The listing builds one solid part. Answer for the finished solid, in the listing's coordinates (mm). Face numbers are marked on the shaded views. Round coordinates to 2 decimals unless told otherwise and drop trailing zeros. Write each loop counter-clockwise with the first axis right and the second up, starting at its lowest first coordinate (ties: lowest second). Pieces come first, ordered by that corner, then holes.
Item 1: Each of these flat-tipped pins is pushed along its axis until it touches: pin 1 (1.5 mm diameter, centred on y = 12.5, z = 15, fed in from -X); pin 2 (3 mm diameter, centred on x = -8, z = -44.5, fed in from +Y); pin 3 (12 mm diameter, centred on x = 11, z = 60.5, fed in from +Y). Where does it stop, or does it pass through?
Item 2: For a pull along X with two mould halves and no side action, classify the marked faces 1 and 2 as +X half, -X half, draft (parallel to the pull), parting line (faces both ways), or undercut.
Item 3: Find section A-A on x = 0. Give the vertices of the cut face in (y, z), then the cut area to 3 significant figures.
Item 4: Find the intervals of material crossed by probe 1 along Z at (x, y) = (0, 13); probe 2 along Y at (x, z) = (0, 21); probe 3 along Z at (x, y) = (-1.5, 12), in increasing order.
Item 5: Find section C-C on z = -13. Give the vertices of the cut face in (x, y).
Item 6: Find section D-D on y = -4. Give the vertices of the cut face in (x, z).
Item 7: Find section B-B on y = 3.5. Give the vertices of the cut face in (x, z).
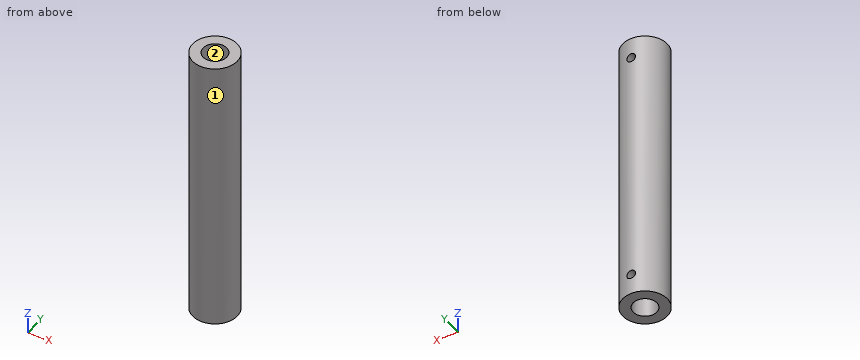
```python
from build123d import *

# Parameters (mm, degrees)
SKETCH2_R                = 16
SKETCH2_R_2              = 8.5
BOSS_EXTRUDE1_DEPTH      = 100
BOSS_EXTRUDE1_DEPTH_BACK = 100
SKETCH4_R                = 3.1
CUT_EXTRUDE1_DEPTH       = 17


with BuildPart() as part:
    # Sketch2 → Boss-Extrude1 (new body, two sides)
    with BuildSketch(Plane.XY) as boss_extrude1_sk:
        Circle(SKETCH2_R)
        Circle(SKETCH2_R_2, mode=Mode.SUBTRACT)
    extrude(amount=BOSS_EXTRUDE1_DEPTH)
    extrude(boss_extrude1_sk.sketch, amount=-BOSS_EXTRUDE1_DEPTH_BACK)

    # Sketch4 → Cut-Extrude1 (cut, through all)
    with BuildSketch(Plane(origin=(0, 0, 0), x_dir=(1, 0, 0), z_dir=(0, 1, 0))):
        with Locations((0, -85)):
            Circle(SKETCH4_R)
    cut_extrude1 = extrude(amount=CUT_EXTRUDE1_DEPTH, mode=Mode.SUBTRACT)

    # Mirror1: Cut-Extrude1 across plane
    add(cut_extrude1.mirror(Plane.XY), mode=Mode.SUBTRACT)


solid = part.part
```
Check values:
1. pin 1: stops at x = -10.86
1. pin 2: stops at y = 14.62
1. pin 3: stops at y = 15.2
2. face 1: parting line
2. face 2: undercut
3. outline: (-16, -100) - (-8.5, -100) - (-8.5, 100) - (-16, 100) - close; (8.5, -100) - (16, -100) - (16, -88.1) - (8.5, -88.1) - close; (8.5, -81.9) - (16, -81.9) - (16, 81.9) - (8.5, 81.9) - close; (8.5, 88.1) - (16, 88.1) - (16, 100) - (8.5, 100) - close
3. area: 2,910 mm2
4. probe 1: z = -100 to -88.1, -81.9 to 81.9, 88.1 to 100
4. probe 2: y = -16 to -8.5, 8.5 to 16
4. probe 3: z = -100 to -87.71, -82.29 to 82.29, 87.71 to 100
5. outline: circle Ø32 at (0, 0); hole circle Ø17 at (0, 0)
6. outline: (-15.49, -100) - (-7.5, -100) - (-7.5, 100) - (-15.49, 100) - close; (7.5, -100) - (15.49, -100) - (15.49, 100) - (7.5, 100) - close
7. outline: (-15.61, -100) - (-7.75, -100) - (-7.75, 100) - (-15.61, 100) - close; (7.75, -100) - (15.61, -100) - (15.61, 100) - (7.75, 100) - close
